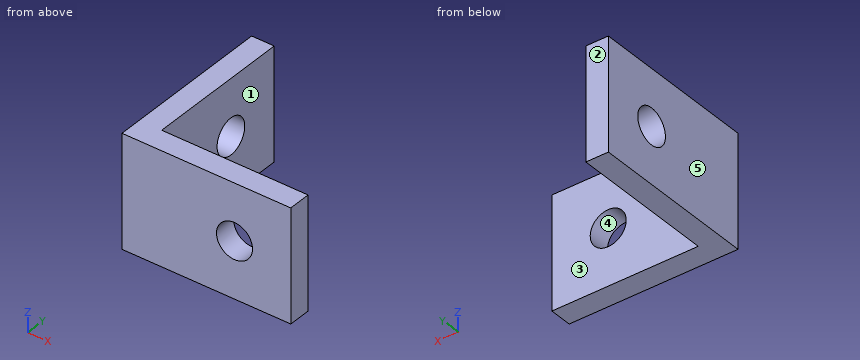
from build123d import *

# Parameters (mm, degrees)
BASE_DEPTH                       = 5
F_3_2_3_2_MOUNTHOLES_D           = 3.2
F_3_2_3_2_MOUNTHOLES_ON_FACE_2_D = 3.2


with BuildPart() as part:
    # Sketch1 → Base (new body, symmetric)
    with BuildSketch(Plane.XY):
        Polygon((0, 0), (0, 15), (2, 15), (2, 2), (15, 2), (15, 0), align=None)
    extrude(amount=BASE_DEPTH, both=True)

    # Ø3.2 (3.2) MountHoles (through all)
    with Locations(Plane(origin=(0, 10, 0), x_dir=(0, 0, -1), z_dir=(-1, 0, 0))):
        with Locations((0, 0)):
            Hole(F_3_2_3_2_MOUNTHOLES_D / 2)

    # Ø3.2 (3.2) MountHoles on face 2 (through all)
    with Locations(Plane(origin=(10, 0, 0), x_dir=(0, 0, -1), z_dir=(0, -1, 0))):
        with Locations((0, 0)):
            Hole(F_3_2_3_2_MOUNTHOLES_ON_FACE_2_D / 2)


solid = part.part
Can you work these out from the model? Positions are in its coordinate system, mm. Face numbers are marked on the shaded views. A direction names the side the tool comes from. Give positions to 0.01 mm unless a question says otherwise; leave off trailing zeros. Loops run counter-clockwise (first coordinate to the right, second up) from the corner with the lowest first, then second, coordinate; pieces in that order, holes last. Notation, with made-up numbers: (20.5, 15) - (64.5, 15) arc R13 cw to (64.5, 25) - close; hole circle Ø8 at (18.25, -28.5). An arc over 180 degrees is marked (long way). One line per item, written item: value.
(1) If we mould it in two halves opening along X, with no side actions, what happens to the marked faces 3, 4 and 5? For each: released by +X, released by -X, zero draft, split by the parting line, or undercut.
Verdict:
face 3: zero draft
face 4: undercut
face 5: released by -X
(2) On a 3-axis mill with a long thin cutter (end or side, diameter ignored), from which of +Z, -Z, +X, -X, +Y, -Y can I reach the whole of each face in a straight line? I mean the marked faces 1 and 2. Say none if no direction works.
Verdict:
face 1: +Z, -Z, +X, +Y
face 2: +Z, -Z, +X, -X, +Y
(3) If we section it at A-A, the plane z = 0: List the corners of the cut face in (x, y) for me, plus the area to 3 significant figures.
Verdict:
outline: (0, 0) - (8.4, 0) - (8.4, 2) - (2, 2) - (2, 8.4) - (0, 8.4) - close; (0, 11.6) - (2, 11.6) - (2, 15) - (0, 15) - close; (11.6, 0) - (15, 0) - (15, 2) - (11.6, 2) - close
area: 43.2 mm^2
(4) I need wall thicknesses on line 1 along X through (y, z) = (1.2, 0); line 2 along Z through (x, y) = (0.8, 10); line 3 along Y through (x, z) = (12.25, -2). Which ranges of each line are inside material? Lowest first, please.
Verdict:
line 1: 0 to 8.4, 11.6 to 15
line 2: -5 to -1.6, 1.6 to 5
line 3: 0 to 2
(5) If we section it at B-B, the plane x = 10: List the corners of the cut face in (y, z) for me.
Verdict:
outline: (0, -5) - (2, -5) - (2, -1.6) - (0, -1.6) - close; (0, 1.6) - (2, 1.6) - (2, 5) - (0, 5) - close
(6) If we section it at D-D, the plane y = 1.5: List the corners of the cut face in (x, z) for me, plus the area to 3 significant figures.
Verdict:
outline: (0, -5) - (15, -5) - (15, 5) - (0, 5) - close; hole circle Ø3.2 at (10, 0)
area: 142 mm^2
(7) I'm going to push flat-ended pins straight in: pin 1 (4 mm diameter, centred on x = 10, z = 0, fed in from +Y); pin 2 (3.5 mm diameter, centred on y = 10, z = 0, fed in from +X). Where does each tip first touch, or does it pass through?
Verdict:
pin 1: y = 2
pin 2: x = 2
